Part model, mm, in its own coordinate system. Face numbers are marked on the shaded views. A direction names the side the tool comes from. Round coordinates to 2 decimals unless told otherwise and drop trailing zeros. Loops run counter-clockwise (first coordinate to the right, second up) from the corner with the lowest first, then second, coordinate; pieces in that order, holes last.
from build123d import *

# Parameters (mm, degrees)
SKETCH2_R           = 2.6
BOSS_EXTRUDE1_DEPTH = 1
CUT_EXTRUDE1_DEPTH  = 0.6


with BuildPart() as part:
    # Sketch2 → Boss-Extrude1 (new body)
    with BuildSketch(Plane.XY):
        Polygon((-6.3, 10.3), (-6.3, -10.3), (-5.3, -10.3), (6.3, -10.3), (8.1, -10.3), (12.9, -10.3), (12.9, 10.3), (8.1, 10.3), (6.3, 10.3), (-5.3, 10.3), align=None)
        Circle(SKETCH2_R, mode=Mode.SUBTRACT)
    extrude(amount=BOSS_EXTRUDE1_DEPTH)

    # Sketch3 → Cut-Extrude1 (cut)
    with BuildSketch(Plane.XY):
        Polygon((5.3, 8.5), (5.3, -8.5), (6.3, -8.5), (12.9, -8.5), (12.9, 8.5), (6.3, 8.5), align=None)
    extrude(amount=CUT_EXTRUDE1_DEPTH, mode=Mode.SUBTRACT)


solid = part.part
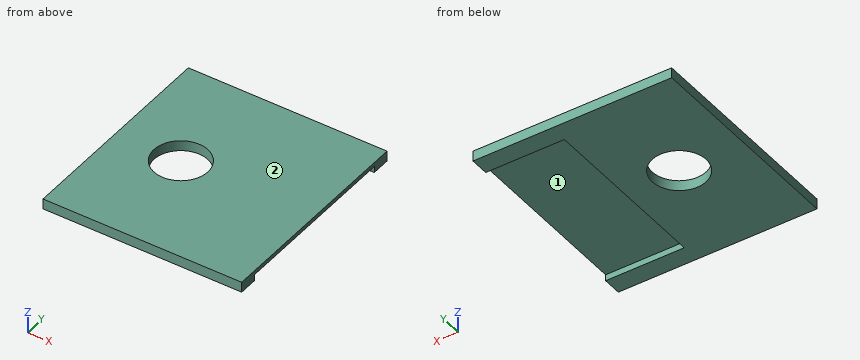
1) Slice it at D-D, the plane x = 11. Give the cut face in (y, z).
Values:
outline: (-10.3, 0) - (-8.5, 0) - (-8.5, 0.6) - (8.5, 0.6) - (8.5, 0) - (10.3, 0) - (10.3, 1) - (-10.3, 1) - close
2) Slice it at A-A, the plane y = 0. Give the cut face in (x, z), then the cut area to 3 significant figures.
Values:
outline: (-6.3, 0) - (-2.6, 0) - (-2.6, 1) - (-6.3, 1) - close; (2.6, 0) - (5.3, 0) - (5.3, 0.6) - (12.9, 0.6) - (12.9, 1) - (2.6, 1) - close
area: 9.44 mm2
3) Tool access for the marked faces 1 and 2: list every direction of +Z, -Z, +X, -X, +Y, -Y with a clear straight run to the whole face (end or side of a thin tool).
Values:
face 1: -Z, +X
face 2: +Z, +X, -X, +Y, -Y
4) Slice it at B-B, the plane z = 0.85. Give the cut face in (x, y), then the cut area to 3 significant figures.
Values:
outline: (-6.3, -10.3) - (12.9, -10.3) - (12.9, 10.3) - (-6.3, 10.3) - close; hole circle Ø5.2 at (0, 0)
area: 374 mm2
5) Slice it at C-C, the plane x = 1.75. Give the cut face in (y, z).
Values:
outline: (-10.3, 0) - (-1.92, 0) - (-1.92, 1) - (-10.3, 1) - close; (1.92, 0) - (10.3, 0) - (10.3, 1) - (1.92, 1) - close
6) Wall check: line 1 along Y through (x, z) = (0, 0.85); line 2 along Y through (x, z) = (5.5, 0.5); line 3 along Z through (x, y) = (11, -2.5). Give the ranges that are in metal, low to high.
Values:
line 1: y = -10.3 to -2.6, 2.6 to 10.3
line 2: y = -10.3 to -8.5, 8.5 to 10.3
line 3: z = 0.6 to 1
7) Drop flat-ended pins along their axis: pin 1 Ø4 at (x, y) = (8.5, -2) entering from -Z; pin 2 Ø8 at (x, y) = (-2, -5) entering from -Z. Give the stop position or say it passes through.
Values:
pin 1: stops at z = 0.6
pin 2: stops at z = 0
